Verification items for the finished model (mm, model axes). A direction names the side the tool comes from. Round coordinates to 2 decimals unless told otherwise and drop trailing zeros. Loops run counter-clockwise (first coordinate to the right, second up) from the corner with the lowest first, then second, coordinate; pieces in that order, holes last. Notation, with made-up numbers: (-19.5, 6.25) - (14.5, 6.25) arc R33 ccw to (14.5, 43.25) - close; hole circle Ø7 at (-33.5, 46). An arc over 180 degrees is marked (long way). Use CSV: the item, a comma, the result in double quotes.
```python
from build123d import *

# Parameters (mm, degrees)
SKETCH012_R     = 2
PAD010_DEPTH    = 10
SKETCH013_R     = 3
POCKET_DEPTH    = 2.5
SKETCH014_R     = 3
POCKET001_DEPTH = 2.5


with BuildPart() as part:
    # Sketch012 → Pad010 (new body)
    with BuildSketch(Plane.XZ.offset(-20)):
        with BuildLine():
            Line((-11.287198, -7.55), (-5.196164, 2.99998))
            ThreePointArc((5.196164, 2.99998), (0, 6), (-5.196164, 2.99998))
            Line((5.196164, 2.99998), (11.287198, -7.55))
            Line((11.287198, -7.55), (-11.287198, -7.55))
        make_face()
        Circle(SKETCH012_R, mode=Mode.SUBTRACT)
    extrude(amount=PAD010_DEPTH)

    # Sketch013 → Pocket (cut)
    with BuildSketch(Plane.XZ.offset(-10)):
        Circle(SKETCH013_R)
    extrude(amount=-POCKET_DEPTH, mode=Mode.SUBTRACT)

    # Sketch014 → Pocket001 (cut)
    with BuildSketch(Plane(origin=(0, 20, 0), x_dir=(1, 0, 0), z_dir=(0, 1, 0))):
        Circle(SKETCH014_R)
    extrude(amount=-POCKET001_DEPTH, mode=Mode.SUBTRACT)


solid = part.part
```
1) Cross-section at A-A, the plane x = 0. Record the cut outline in (y, z), then the cut area to 3 significant figures.
Returned:
outline,"(10, -7.55) - (20, -7.55) - (20, -3) - (17.5, -3) - (17.5, -2) - (12.5, -2) - (12.5, -3) - (10, -3) - close; (10, 3) - (12.5, 3) - (12.5, 2) - (17.5, 2) - (17.5, 3) - (20, 3) - (20, 6) - (10, 6) - close"
area,"85.5 mm²"
2) Access from +Z, -Z, +X, -X, +Y, -Y to the whole of each face (thin tool, end or side, straight path). Record for faces 1 (the face through (-3, 19, 0)), 2 (the face through (0, 15, -7.55)), 3 (the face through (1, 12.5, -2)).
Returned:
face 1,"+Y"
face 2,"-Z, +X, -X, +Y, -Y"
face 3,"-Y"
3) Cross-section at D-D, the plane y = 14.5. Record the cut outline in (x, z), then the cut area to 3 significant figures.
Returned:
outline,"(-11.29, -7.55) - (11.29, -7.55) - (5.2, 3) arc R6 ccw to (-5.2, 3) - close; hole circle Ø4 at (0, 0)"
area,"183 mm²"
4) Gauge pin test, flat ends, axial feed: pin 1 Ø5 at (y, z) = (11.5, 1) entering from -X; pin 2 Ø1.5 at (y, z) = (16.5, 0) entering from -X; pin 3 Ø2 at (y, z) = (16.5, -1.5) entering from -X. Record the tip position at first contact, or that the pin passes through.
Returned:
pin 1,"stops at x = -7.79"
pin 2,"stops at x = -7.36"
pin 3,"stops at x = -8.37"
5) Cross-section at C-C, the plane z = 0. Record the cut outline in (x, y).
Returned:
outline,"(-6.93, 10) - (-3, 10) - (-3, 12.5) - (-2, 12.5) - (-2, 17.5) - (-3, 17.5) - (-3, 20) - (-6.93, 20) - close; (2, 12.5) - (3, 12.5) - (3, 10) - (6.93, 10) - (6.93, 20) - (3, 20) - (3, 17.5) - (2, 17.5) - close"
6) Thickness scan on probe 1 along X at (y, z) = (19.75, 1.75); probe 2 along X at (y, z) = (19, 0); probe 3 along Y at (x, z) = (1.75, -1.5). Record the ranges inside material, lowest first. Write a range as [from, to].
Returned:
probe 1,"x = [-5.92, -2.44], [2.44, 5.92]"
probe 2,"x = [-6.93, -3], [3, 6.93]"
probe 3,"y = [12.5, 17.5]"
7) Cross-section at B-B, the plane y = 11.75. Record the cut outline in (x, z), then the cut area to 3 significant figures.
Returned:
outline,"(-11.29, -7.55) - (11.29, -7.55) - (5.2, 3) arc R6 ccw to (-5.2, 3) - close; hole circle Ø6 at (0, 0)"
area,"168 mm²"
